from build123d import *

# Parameters (mm, degrees)
SKIZZE1_W                        = 35
SKIZZE1_H                        = 75
AUFSATZ_LINEAR_AUSTRAGEN1_DEPTH  = 1.5
SKIZZE3_W                        = 15.25
SKIZZE3_H                        = 5
SKIZZE3_W_2                      = 4.875
SCHNITT_LINEAR_AUSTRAGEN12_DEPTH = 20
SKIZZE13_R                       = 12
SCHNITT_LINEAR_AUSTRAGEN18_DEPTH = 1.5
SKIZZE14_W                       = 1
SKIZZE14_H                       = 57.312152727
AUFSATZ_LINEAR_AUSTRAGEN8_DEPTH  = 1.5


with BuildPart() as part:
    # Skizze1 → Aufsatz-Linear austragen1 (new body)
    with BuildSketch(Plane.XY):
        with Locations((17.5, 37.5)):
            Rectangle(SKIZZE1_W, SKIZZE1_H)
    extrude(amount=AUFSATZ_LINEAR_AUSTRAGEN1_DEPTH)

    # Skizze3 → Schnitt-Linear austragen12 (cut)
    with BuildSketch(Plane.XY.offset(1.5)):
        with Locations((17.5, 2.5)):
            Rectangle(SKIZZE3_W, SKIZZE3_H)
        with Locations((32.5625, 2.5)):
            Rectangle(SKIZZE3_W_2, SKIZZE3_H)
        with Locations((2.4375, 2.5)):
            Rectangle(SKIZZE3_W_2, SKIZZE3_H)
    extrude(amount=-SCHNITT_LINEAR_AUSTRAGEN12_DEPTH, mode=Mode.SUBTRACT)

    # Skizze13 → Schnitt-Linear austragen18 (cut)
    with BuildSketch(Plane.XY.offset(1.5)):
        with BuildLine():
            Line((14.905768525, 40.7415201), (14.913283553, 40.740050943))
            ThreePointArc((14.913283553, 40.740050943), (17.550982946, 15.000099972), (19.986710673, 40.759947885))
            ThreePointArc((19.986710673, 40.759947885), (17.352851338, 66.4999145), (14.905768525, 40.7415201))
        make_face()
        with Locations((17.4, 53.5)):
            Circle(SKIZZE13_R, mode=Mode.SUBTRACT)
        with Locations((17.5, 28)):
            Circle(SKIZZE13_R, mode=Mode.SUBTRACT)
    extrude(amount=-SCHNITT_LINEAR_AUSTRAGEN18_DEPTH, mode=Mode.SUBTRACT)


with BuildPart() as schnitt_linear_austragen18_piece_1:
    # of the separate pieces the step leaves, piece 1, a body of its own (schnitt_linear_austragen18_pieces)
    add(part.part.solids().sort_by_distance((4.875, 0, 0))[0])



with BuildPart() as schnitt_linear_austragen18_piece_2:
    # of the separate pieces the step leaves, piece 2, a body of its own (schnitt_linear_austragen18_pieces)
    add(part.part.solids().sort_by_distance((29.4, 53.5, 0))[0])


with BuildPart() as schnitt_linear_austragen18_piece_3:
    # of the separate pieces the step leaves, piece 3, a body of its own (schnitt_linear_austragen18_pieces)
    add(part.part.solids().sort_by_distance((29.5, 28, 0))[0])


with BuildPart() as schnitt_linear_austragen18_piece_1_1:
    add(schnitt_linear_austragen18_piece_1.part)

    add(schnitt_linear_austragen18_piece_2.part)  # Aufsatz-Linear austragen8 merges Schnitt-Linear austragen18 piece 2

    add(schnitt_linear_austragen18_piece_3.part)  # Aufsatz-Linear austragen8 merges Schnitt-Linear austragen18 piece 3
    # Skizze14 → Aufsatz-Linear austragen8 (add)
    with BuildSketch(Plane.XY.offset(1.5)):
        with Locations((17.5, 39.529651928)):
            Rectangle(SKIZZE14_W, SKIZZE14_H)
    extrude(amount=-AUFSATZ_LINEAR_AUSTRAGEN8_DEPTH)


solid = schnitt_linear_austragen18_piece_1_1.part
Part model, mm, in its own coordinate system. A direction names the side the tool comes from. Coordinates: 2 decimals unless noted, no trailing zeros. Loops run counter-clockwise (first coordinate to the right, second up) from the corner with the lowest first, then second, coordinate; pieces in that order, holes last. Notation, with made-up numbers: M 87,53.25 L 95,53.25 A22 ccw 95,77.25 Z; hole C 63,30 d4. An arc over 180 degrees is marked long. Use a Markdown table: item, result. Add a question column.
Q1. Cut at B-B (x = 26). Write the cut outline in (y, z), and give its area (3 significant figures).
Q2. Mould opens along X. For faces 1 (the flat face through (18, 41, 1)), 2 (the cylindrical face through (30.44, 26.74, 0.76)), 3 (the flat face through (2, 5, 1)), 4 (the flat face through (0, 40, 1)) say: +X half, -X half, draft (parallel to the pull), parting line (faces both ways), or undercut.
Q3. Cut at A-A (y = 53.5). Write the cut outline in (x, z).
Q4. Cut at D-D (y = 64). Write the cut outline in (x, z).
Q5. Which spindle directions (+Z, -Z, +X, -X, +Y, -Y) get a long thin tool onto all of the face, cutting with end or side? Do faces 5 (the flat face through (28, 0, 1)), 6 (the cylindrical face through (29.397, 53.245, 0.76)), 7 (the flat face through (17, 38, 0)), 8 (the flat face through (17, 5, 1)), 9 (the flat face through (33, 5, 1)). Say none if no direction does.
Q6. Cut at C-C (z = 1). Write the cut outline in (x, y) (3 decimals).
Q7. Probe L1, parallel to X at y = 3.5, z = 0.9 (3 decimals); L2, parallel to Y at x = 23, z = 1.3; L3, parallel to X at y = 63, z = 1.3. List the from-to ranges inside material, lowest first.
Worked out:
| question | item | result |
|---|---|---|
| 1 | outline | M 0,0 L 18.16,0 L 18.16,1.5 L 0,1.5 Z; M 19.53,0 L 36.47,0 L 36.47,1.5 L 19.53,1.5 Z; M 37.84,0 L 43.75,0 L 43.75,1.5 L 37.84,1.5 Z; M 45.13,0 L 61.87,0 L 61.87,1.5 L 45.13,1.5 Z; M 63.25,0 L 75,0 L 75,1.5 L 63.25,1.5 Z |
| 1 | area | 104 mm2 |
| 2 | face 1 | undercut |
| 2 | face 2 | undercut |
| 2 | face 3 | draft |
| 2 | face 4 | -X half |
| 3 | outline | M 0,0 L 4.4,0 L 4.4,1.5 L 0,1.5 Z; M 5.4,0 L 29.4,0 L 29.4,1.5 L 5.4,1.5 Z; M 30.4,0 L 35,0 L 35,1.5 L 30.4,1.5 Z |
| 4 | outline | M 0,0 L 9.74,0 L 9.74,1.5 L 0,1.5 Z; M 11.59,0 L 23.21,0 L 23.21,1.5 L 11.59,1.5 Z; M 25.06,0 L 35,0 L 35,1.5 L 25.06,1.5 Z |
| 5 | face 5 | +Z, -Z, +X, -X, -Y |
| 5 | face 6 | +Z, -Z |
| 5 | face 7 | -Z, +X, -X, +Y, -Y |
| 5 | face 8 | +Z, -Z, -Y |
| 5 | face 9 | +Z, -Z, +X, -Y |
| 6 | outline | M 0,5 L 4.875,5 L 4.875,0 L 9.875,0 L 9.875,5 L 25.125,5 L 25.125,0 L 30.125,0 L 30.125,5 L 35,5 L 35,75 L 0,75 Z; hole M 14.906,40.742 L 14.913,40.74 A13 ccw 17,15.01 L 17,16.01 A12 cw 17,39.99 L 17,41.507 A12 cw 17,65.493 L 17,66.494 A13 ccw Z; hole M 18,15.01 A13 ccw 19.987,40.76 A13 ccw 18,66.486 L 18,65.485 A12 cw 18,41.515 L 18,39.99 A12 cw 18,16.01 Z |
| 7 | L1 | x = 4.875 to 9.875, 25.125 to 30.125 |
| 7 | L2 | y = 5 to 16.22, 17.33 to 38.67, 39.78 to 41.77, 42.89 to 64.11, 65.23 to 75 |
| 7 | L3 | x = 0 to 8.53, 10.07 to 24.73, 26.27 to 35 |
